For this review, use the dimensioned drawing (mm, ordinates from the lowest corner) and the shaded views. Round coordinates to 2 decimals unless told otherwise and drop trailing zeros. Write each loop counter-clockwise with the first axis right and the second up, starting at its lowest first coordinate (ties: lowest second). Pieces come first, ordered by that corner, then holes. Notation, with made-up numbers: M 81,-2 L 135,-2 A8 cw 135,5 Z; hole C 42,-36.5 d8. An arc over 180 degrees is marked long. Use CSV: the item, a comma, the result in double quotes.
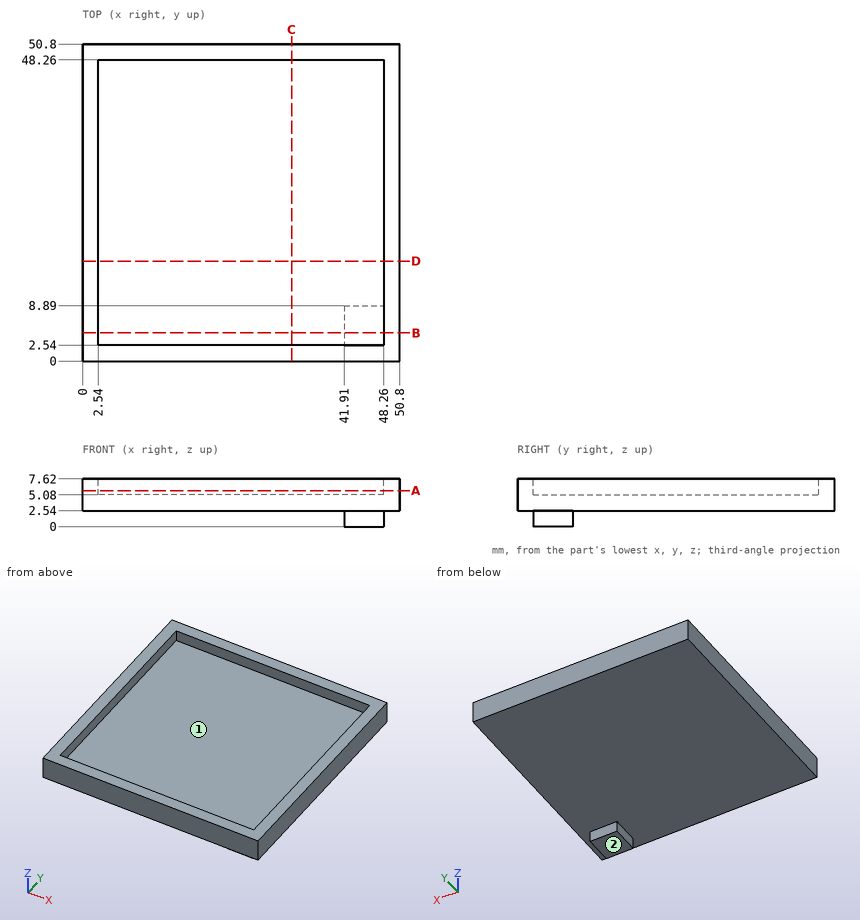
1) Add section B-B on y = 4.5. Write out the cut boundary in (x, z), then the cut area to 3 significant figures.
Answers:
outline,"M 0,2.54 L 41.91,2.54 L 41.91,0 L 48.26,0 L 48.26,2.54 L 50.8,2.54 L 50.8,7.62 L 48.26,7.62 L 48.26,5.08 L 2.54,5.08 L 2.54,7.62 L 0,7.62 Z"
area,"158 mm²"
2) For pin 1 Ø2 at (x, y) = (29, 12.5) entering from -Z; pin 2 Ø1 at (x, y) = (12.5, 14) entering from +Z; pin 3 Ø3 at (x, z) = (45, 1) entering from +Y, all flat-tipped, find the tip position at first contact; note any pin that passes through.
Answers:
pin 1,"z = 2.54"
pin 2,"z = 5.08"
pin 3,"y = 8.89"
3) Add section A-A on z = 5.75. Write out the cut boundary in (x, y), then the cut area to 3 significant figures.
Answers:
outline,"M 0,0 L 50.8,0 L 50.8,50.8 L 0,50.8 Z; hole M 2.54,2.54 L 48.26,2.54 L 48.26,48.26 L 2.54,48.26 Z"
area,"490 mm²"
4) Wall thickness on line 1 along X through (y, z) = (36, 5.5); line 2 along Z through (x, y) = (15.5, 23.5): over which ranges is each line inside the solid? List them lowest first. Write a range as [from, to].
Answers:
line 1,"[0, 2.54], [48.26, 50.8]"
line 2,"[2.54, 5.08]"
5) The part is to be moulded in two halves that separate along X. For the marked faces 1 and 2, say which applies: released by +X, released by -X, zero draft, split by the parting line, or undercut.
Answers:
face 1,"undercut"
face 2,"zero draft"
6) Add section C-C on x = 33.5. Write out the cut boundary in (y, z).
Answers:
outline,"M 0,2.54 L 50.8,2.54 L 50.8,7.62 L 48.26,7.62 L 48.26,5.08 L 2.54,5.08 L 2.54,7.62 L 0,7.62 Z"
